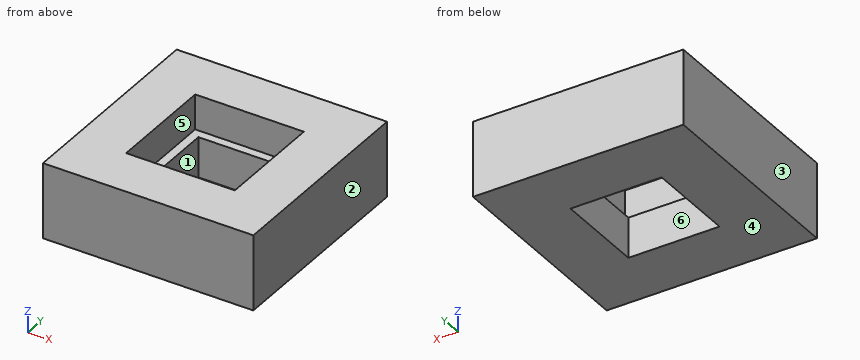
```python
from build123d import *

# Parameters (mm, degrees)
F0_W     = 120
F0_H     = 120
F1_DEPTH = 3
F2_W     = 52
F2_H     = 52
F3_DEPTH = 25
F2_W_2   = 120
F2_H_2   = 120
F2_W_3   = 70
F2_H_3   = 70
F2_R     = 2.5
F4_DEPTH = 37
F5_W     = 120
F5_H     = 120
F5_W_2   = 114
F5_H_2   = 114
F5_W_3   = 52
F5_H_3   = 52
F6_DEPTH = 3
F7_W     = 62
F7_H     = 62
F7_W_2   = 52
F7_H_2   = 52
F8_DEPTH = 20


with BuildPart() as f1:
    # F0 (on Top) → F1 (new body)
    with BuildSketch(Plane.XY):
        Rectangle(F0_W, F0_H)
    extrude(amount=F1_DEPTH)

    # F2 (on face) → F3 (cut)
    with BuildSketch(Plane.XY.offset(3)):
        Rectangle(F2_W, F2_H)
    extrude(amount=-F3_DEPTH, mode=Mode.SUBTRACT)

    # F2 (on face) → F4 (join)
    with BuildSketch(Plane.XY.offset(3)):
        Rectangle(F2_W_2, F2_H_2)
        Polygon((-57, -57), (-57, -35), (-57, 35), (-57, 57), (-35, 57), (35, 57), (57, 57), (57, 35), (57, -35), (57, -57), (35, -57), (-35, -57), align=None, mode=Mode.SUBTRACT)
        Rectangle(F2_W_3, F2_H_3)
        Rectangle(F2_W, F2_H, mode=Mode.SUBTRACT)
        with Locations((46, 46)):
            Circle(F2_R)
        with Locations((0, 46)):
            Circle(F2_R)
        with Locations((-46, 46)):
            Circle(F2_R)
        with Locations((-46, 0)):
            Circle(F2_R)
        with Locations((-46, -46)):
            Circle(F2_R)
        with Locations((0, -46)):
            Circle(F2_R)
        with Locations((46, -46)):
            Circle(F2_R)
        with Locations((46, 0)):
            Circle(F2_R)
    extrude(amount=F4_DEPTH)

    # F5 (on face) → F6 (join)
    with BuildSketch(Plane.XY.offset(40)):
        Rectangle(F5_W, F5_H)
        Rectangle(F5_W_2, F5_H_2, mode=Mode.SUBTRACT)
        Rectangle(F5_W_2, F5_H_2)
        Rectangle(F5_W_3, F5_H_3, mode=Mode.SUBTRACT)
    extrude(amount=F6_DEPTH)

    # F7 (on face) → F8 (cut)
    with BuildSketch(Plane.XY.offset(43)):
        Rectangle(F7_W, F7_H)
        Rectangle(F7_W_2, F7_H_2, mode=Mode.SUBTRACT)
    extrude(amount=-F8_DEPTH, mode=Mode.SUBTRACT)


solid = f1.part
```
Model file for the job. Use its own axes, mm. Face numbers are marked on the shaded views. A direction names the side the tool comes from. Give positions to 0.01 mm unless a question says otherwise; leave off trailing zeros. Order: outer loops, then holes, each group sorted by start corner. A loop starts at its lowest first (then second) coordinate and runs counter-clockwise, first axis right, second up.
1) Saw through at C-C, the plane z = 24.5. Count the separate pieces of the cut face and the enclosed holes in it, then the cut area to 3 significant figures.
2) Wall check: probe 1 along Y at (x, z) = (18, 26.5); probe 2 along Y at (x, z) = (6.5, 5). Give the ranges that are in metal, low to high.
3) Saw through at A-A, the plane x = 8. Write the cut outline in (y, z).
4) 3-axis set-ups, long thin cutter, end or side, ignore diameter. For the marked faces 4, 5 and 6: which of +Z, -Z, +X, -X, +Y, -Y reach the whole face in a straight line?
5) Mould opens along X. For the marked faces 1, 2 and 3 say: +X half, -X half, draft (parallel to the pull), parting line (faces both ways), or undercut.
6) Saw through at D-D, the plane y = 0. Write the cut outline in (x, z), then the cut area to 3 significant figures.
Computed:
1. separate pieces: 10
1. enclosed holes: 2
1. area: 2,620 mm2
2. probe 1: y = -60 to -57, -35 to -31, 31 to 35, 57 to 60
2. probe 2: y = -60 to -57, -35 to -26, 26 to 35, 57 to 60
3. outline: (-60, 0) - (-26, 0) - (-26, 23) - (-31, 23) - (-31, 43) - (-60, 43) - close; (26, 0) - (60, 0) - (60, 43) - (31, 43) - (31, 23) - (26, 23) - close; hole (-57, 3) - (-35, 3) - (-35, 40) - (-57, 40) - close; hole (35, 3) - (57, 3) - (57, 40) - (35, 40) - close
4. face 4: -Z, +X, -X, +Y, -Y
4. face 5: +Z
4. face 6: +Z, -Z
5. face 1: undercut
5. face 2: +X half
5. face 3: -X half
6. outline: (-60, 0) - (-26, 0) - (-26, 23) - (-31, 23) - (-31, 43) - (-60, 43) - close; (26, 0) - (60, 0) - (60, 43) - (31, 43) - (31, 23) - (26, 23) - close; hole (-57, 3) - (-48.5, 3) - (-48.5, 40) - (-57, 40) - close; hole (-43.5, 3) - (-35, 3) - (-35, 40) - (-43.5, 40) - close; hole (35, 3) - (43.5, 3) - (43.5, 40) - (35, 40) - close; hole (48.5, 3) - (57, 3) - (57, 40) - (48.5, 40) - close
6. area: 1,470 mm2
